from build123d import *

# Parameters (mm, degrees)
F0_R     = 2
F1_DEPTH = 2.5
F2_DEPTH = 40
F3_R     = 1.625
F4_DEPTH = 25


# Not quite as in the source:
# - a feature names something its author has since deleted; it is built from what else it names


with BuildPart() as f1:
    # F0 (on Top) → F1 (new body)
    with BuildSketch(Plane.XY):
        Polygon((29.9, 29.9), (-29.9, 29.9), (-29.9, -29.9), (29.9, -29.9), (29.9, 10.2), (1.0269208253, 10.2), (0.8924006252, 10.2), (-0.932000461, 10.2), (-10.1, 10.2), (-10.1, 12.7), (29.9, 12.7), align=None)
        with Locations((-23.9, -23.9)):
            Circle(F0_R, mode=Mode.SUBTRACT)
        with Locations((23.9, -23.9)):
            Circle(F0_R, mode=Mode.SUBTRACT)
        with BuildLine():
            ThreePointArc((1.0269208253, 3.4086703593), (2.8573972543, 2.1234125673), (3.56, 0))
            ThreePointArc((3.56, 0), (-2.1628312878, -2.8276776373), (-0.932000461, 3.4358368909))
            Line((-0.932000461, 3.4358368909), (-0.932000461, 5.8278255165))
            Line((-0.932000461, 5.8278255165), (1.0269208253, 5.8278255165))
            Line((1.0269208253, 5.8278255165), (1.0269208253, 3.4086703593))
        make_face(mode=Mode.SUBTRACT)
        with Locations((-23.9, 23.9)):
            Circle(F0_R, mode=Mode.SUBTRACT)
        with Locations((23.9, 23.9)):
            Circle(F0_R, mode=Mode.SUBTRACT)
    extrude(amount=F1_DEPTH)

    # F0 (on Top) → F2 (join)
    with BuildSketch(Plane.XY):
        Polygon((29.9, 10.2), (29.9, 12.7), (-10.1, 12.7), (-10.1, 10.2), (-0.932000461, 10.2), (0.8924006252, 10.2), (1.0269208253, 10.2), align=None)
    extrude(amount=F2_DEPTH)

    # F3 (on face) → F4 (cut)
    with BuildSketch(Plane.XZ.offset(-10.2)):
        with Locations((-7.5884815305, 32.100006938)):
            Circle(F3_R)
        with Locations((-7.475, 7.375)):
            Circle(F3_R)
        with Locations((27.3884814233, 28.875)):
            Circle(F3_R)
        with Locations((27.275, 7.375)):
            Circle(F3_R)
    extrude(amount=-F4_DEPTH, mode=Mode.SUBTRACT)


solid = f1.part
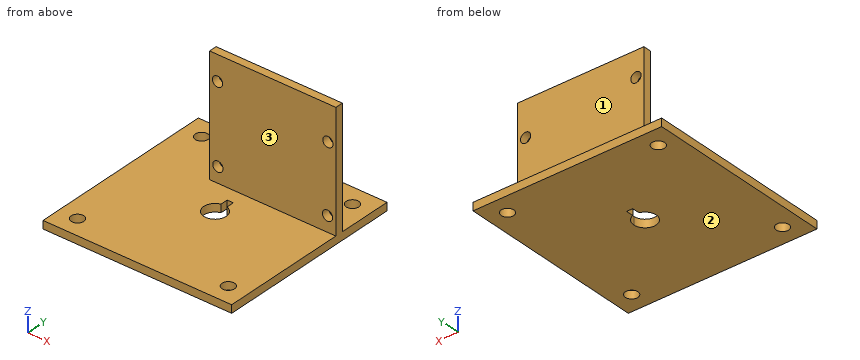
Read the model definition and answer for the solid it produces. Units are mm, in the model's axes. Face numbers are marked on the shaded views. A direction names the side the tool comes from. Coordinates: 2 decimals unless noted, no trailing zeros. Write each loop counter-clockwise with the first axis right and the second up, starting at its lowest first coordinate (ties: lowest second). Pieces come first, ordered by that corner, then holes. Notation, with made-up numbers: (64, 19) -> (113, 19) arc R27 ccw to (113, 44) -> close; hole circle Ø8 at (83, 14.5). An arc over 180 degrees is marked (long way). Return JSON: item names as keys, results as strings.
(1) The part is cut by section A-A on x = 0. Give the vertices of the cut face in (y, z), then the cut area to 3 significant figures.
Answers below:
{"outline": "(-29.9, 0) -> (-3.56, 0) -> (-3.56, 2.5) -> (-29.9, 2.5) -> close; (5.83, 0) -> (29.9, 0) -> (29.9, 2.5) -> (12.7, 2.5) -> (12.7, 40) -> (10.2, 40) -> (10.2, 2.5) -> (5.83, 2.5) -> close", "area": "220 mm^2"}
(2) The part is cut by section B-B on x = -23.9. Give the vertices of the cut face in (y, z), then the cut area to 4 significant figures.
Answers below:
{"outline": "(-29.9, 0) -> (-25.9, 0) -> (-25.9, 2.5) -> (-29.9, 2.5) -> close; (-21.9, 0) -> (21.9, 0) -> (21.9, 2.5) -> (-21.9, 2.5) -> close; (25.9, 0) -> (29.9, 0) -> (29.9, 2.5) -> (25.9, 2.5) -> close", "area": "129.5 mm^2"}
(3) Which of the six approach directions +Z, -Z, +X, -X, +Y, -Y give full straight-line access (tool end or side, diameter ignored) to the marked faces 1, 2 and 3?
Answers below:
{"face 1": "+Z, +X, -X, +Y", "face 2": "-Z, +X, -X, +Y, -Y", "face 3": "+Z, +X, -X, -Y"}
(4) Consider line 1 along Y through (x, z) = (23.9, 0.85); line 2 along X through (y, z) = (-23, 1); line 3 along Z through (x, y) = (-25, 21). Determine where each line is inside the solid, lowest interval first. Write a range as from..to.
Answers below:
{"line 1": "-29.9..-25.9, -21.9..21.9, 25.9..29.9", "line 2": "-29.9..-25.69, -22.11..22.11, 25.69..29.9", "line 3": "0..2.5"}
(5) Each of these flat-tipped pins is pushed along its axis until it touches: P1, Ø3.5, axis at x = -23.9, y = 23.9, coming from the +Z side; P2, Ø2, axis at x = 21.5, y = -13.5, coming from the +Z side; P3, Ø5, axis at x = 27.39, z = 28.88, coming from the +Y side; P4, Ø6, axis at x = -1.5, z = 30, coming from the -Y side. Where does it stop, or does it pass through?
Answers below:
{"P1": "through", "P2": "z = 2.5", "P3": "y = 12.7", "P4": "y = 10.2"}
(6) The part is cut by section D-D on z = 28. Give the vertices of the cut face in (x, y), then the cut area to 3 significant figures.
Answers below:
{"outline": "(-10.1, 10.2) -> (26.02, 10.2) -> (26.02, 12.7) -> (-10.1, 12.7) -> close; (28.76, 10.2) -> (29.9, 10.2) -> (29.9, 12.7) -> (28.76, 12.7) -> close", "area": "93.2 mm^2"}
